```python
from build123d import *

# Parameters (mm, degrees)
SKETCH1_R           = 203.2
SKETCH1_R_2         = 190.5
BOSS_EXTRUDE1_DEPTH = 450
SKETCH2_R           = 323.85
SKETCH2_R_2         = 190.5
SKETCH2_R_3         = 17.5
BOSS_EXTRUDE2_DEPTH = 88.9


with BuildPart() as part:
    # Sketch1 → Boss-Extrude1 (new body)
    with BuildSketch(Plane(origin=(0, 0, 0), x_dir=(1, 0, 0), z_dir=(0, 1, 0))):
        with Locations(Location((0, 0, 0), (0, 0, 270))):
            Circle(SKETCH1_R)
        with Locations(Location((0, 0, 0), (0, 0, 270))):
            Circle(SKETCH1_R_2, mode=Mode.SUBTRACT)
    extrude(amount=BOSS_EXTRUDE1_DEPTH)

    # Sketch2 → Boss-Extrude2 (add)
    with BuildSketch(Plane.XY):
        Circle(SKETCH2_R)
        Circle(SKETCH2_R_2, mode=Mode.SUBTRACT)
        with Locations((285.75, 0)):
            Circle(SKETCH2_R_3, mode=Mode.SUBTRACT)
        with Locations((268.25, 88.301606143)):
            Circle(SKETCH2_R_3, mode=Mode.SUBTRACT)
        with Locations((231.176606143, 167.959635843)):
            Circle(SKETCH2_R_3, mode=Mode.SUBTRACT)
        with Locations(Location((167.959635843, 231.176606143, 0), (0, 0, 271.718815258))):
            Circle(SKETCH2_R_3, mode=Mode.SUBTRACT)
        with Locations((88.301606143, 271.764399531)):
            Circle(SKETCH2_R_3, mode=Mode.SUBTRACT)
        with Locations((0, 289.264399531)):
            Circle(SKETCH2_R_3, mode=Mode.SUBTRACT)
        with Locations((-88.301606143, 271.764399531)):
            Circle(SKETCH2_R_3, mode=Mode.SUBTRACT)
        with Locations(Location((-167.959635843, 231.176606143, 0), (0, 0, 91.718815258))):
            Circle(SKETCH2_R_3, mode=Mode.SUBTRACT)
        with Locations((-231.176606143, 167.959635843)):
            Circle(SKETCH2_R_3, mode=Mode.SUBTRACT)
        with Locations((-271.764399531, 88.301606143)):
            Circle(SKETCH2_R_3, mode=Mode.SUBTRACT)
        with Locations((-289.264399531, 0)):
            Circle(SKETCH2_R_3, mode=Mode.SUBTRACT)
        with Locations((-271.764399531, -88.301606143)):
            Circle(SKETCH2_R_3, mode=Mode.SUBTRACT)
        with Locations((-231.176606143, -167.959635843)):
            Circle(SKETCH2_R_3, mode=Mode.SUBTRACT)
        with Locations((-167.959635843, -231.176606143)):
            Circle(SKETCH2_R_3, mode=Mode.SUBTRACT)
        with Locations((-88.301606143, -271.764399531)):
            Circle(SKETCH2_R_3, mode=Mode.SUBTRACT)
        with Locations((0, -289.264399531)):
            Circle(SKETCH2_R_3, mode=Mode.SUBTRACT)
        with Locations((88.301606143, -271.764399531)):
            Circle(SKETCH2_R_3, mode=Mode.SUBTRACT)
        with Locations((167.959635843, -231.176606143)):
            Circle(SKETCH2_R_3, mode=Mode.SUBTRACT)
        with Locations((231.176606143, -167.959635843)):
            Circle(SKETCH2_R_3, mode=Mode.SUBTRACT)
        with Locations((268.25, -88.301606143)):
            Circle(SKETCH2_R_3, mode=Mode.SUBTRACT)
    extrude(amount=BOSS_EXTRUDE2_DEPTH)


solid = part.part
```
Input: part model. Units: mm. Frame: model coordinates. A direction names the side the tool comes from. Give positions to 0.01 mm unless a question says otherwise; leave off trailing zeros. Order: outer loops, then holes, each group sorted by start corner. A loop starts at its lowest first (then second) coordinate and runs counter-clockwise, first axis right, second up.
1. Line query: probe 1 along Y at (x, z) = (278.5, 45); probe 2 along Y at (x, z) = (-172, 60.5); probe 3 along Y at (x, z) = (140, 67). Output: solid intervals per line, ascending.
Computed:
probe 1: y = -165.28 to -102.49, -74.12 to -15.93, 15.93 to 74.12, 102.49 to 165.28
probe 2: y = -274.4 to -248.2, -214.15 to -81.89, 81.89 to 214.15, 248.2 to 274.4
probe 3: y = -292.03 to -129.19, 129.19 to 292.03
2. Cut plane B-B (y = -135.5). Return loops of the section in (x, z).
Computed:
outline: (-294.14, 0) - (-133.9, 0) - (-133.9, 88.9) - (-294.14, 88.9) - close; (133.9, 0) - (294.14, 0) - (294.14, 88.9) - (133.9, 88.9) - close
3. Pin query (flat end, axial travel): pin 1 Ø10 at (x, y) = (-156, 303) entering from +Z; pin 2 Ø5 at (x, y) = (46, 158) entering from +Z; pin 3 Ø1 at (x, y) = (-111.5, -172) entering from +Z. Return the tip coordinate at first contact, or that it passes through.
Computed:
pin 1: stops at z = 135.98
pin 2: stops at z = 198.49
pin 3: stops at z = 88.9
4. Cut plane C-C (z = -106). Return loops of the section in (x, y).
Computed:
outline: (-173.36, 0) - (-158.29, 0) - (-158.29, 450) - (-173.36, 450) - close; (158.29, 0) - (173.36, 0) - (173.36, 450) - (158.29, 450) - close
5. Draft query along Z for faces 5 (the face through (-2.278, 306.615, 43.828)), 6 (the face through (-289.247, 89.071, 43.828)), 7 (the face through (-5, -224, 0)). Return one class per face: released by +Z, released by -Z, zero draft, split by the parting line, or undercut.
Computed:
face 5: undercut
face 6: zero draft
face 7: released by -Z
6. Cut plane D-D (x = -94). Return loops of the section in (y, z).
Computed:
outline: (-309.91, 0) - (-288.31, 0) - (-288.31, 88.9) - (-309.91, 88.9) - close; (-255.22, 0) - (-165.69, 0) - (-165.69, 88.9) - (-255.22, 88.9) - close; (0, -180.15) - (450, -180.15) - (450, -165.69) - (0, -165.69) - close; (0, 165.69) - (450, 165.69) - (450, 180.15) - (0, 180.15) - close; (165.69, 0) - (255.22, 0) - (255.22, 88.9) - (165.69, 88.9) - close; (288.31, 0) - (309.91, 0) - (309.91, 88.9) - (288.31, 88.9) - close
7. Set-up query: faces 1 (the face through (-59, 450, -182)), 2 (the face through (1, 0, 191)), 3 (the face through (70.82, 272.53, 43.83)), 4 (the face through (1, 0, -192)). Return all of +Z, -Z, +X, -X, +Y, -Y with unobstructed straight access to the full face (end or side cutting, diameter ignored); none if empty.
Computed:
face 1: +Z, -Z, +X, -X, +Y
face 2: +Z, -Z
face 3: none
face 4: -Z, +X, -X, -Y
8. Cut plane A-A (x = 0). Return loops of the section in (y, z), and give its area (3 significant figures).
Computed:
outline: (-323.85, 0) - (-306.76, 0) - (-306.76, 88.9) - (-323.85, 88.9) - close; (-271.76, 0) - (-190.5, 0) - (-190.5, 88.9) - (-271.76, 88.9) - close; (0, -203.2) - (450, -203.2) - (450, -190.5) - (0, -190.5) - close; (0, 190.5) - (450, 190.5) - (450, 203.2) - (0, 203.2) - close; (190.5, 0) - (271.76, 0) - (271.76, 88.9) - (190.5, 88.9) - close; (306.76, 0) - (323.85, 0) - (323.85, 88.9) - (306.76, 88.9) - close
area: 28,900 mm2
